Could you check a few things on this model? Use its own coordinates, in mm. Give positions to 0.01 mm unless a question says otherwise; leave off trailing zeros. Write each loop counter-clockwise with the first axis right and the second up, starting at its lowest first coordinate (ties: lowest second). Pieces come first, ordered by that corner, then holes. Notation, with made-up numbers: (59.5, -24) -> (72.5, -24) arc R23 ccw to (72.5, 6) -> close; hole circle Ø2 at (44, 44). An arc over 180 degrees is marked (long way). One line per question, with ' | ' between items.
from build123d import *

# Parameters (mm, degrees)
BASPROSKE_W         = 20
BASPROSKE_H         = 19.5
TOOTHCUT_DEPTH      = 35.066112194
TEETHCUTS_COUNT     = 11
BORSKE_R            = 2.5
BORE_DEPTH          = 50.0000508
SKETCH1_R           = 2.6
CUT_EXTRUDE1_DEPTH  = 35.008132728
BOSS_EXTRUDE1_DEPTH = 20


with BuildPart() as part:
    # BasProSke → Base-Revolve (revolve)
    with BuildSketch(Plane(origin=(0, 0, 0), x_dir=(1, 0, 0), z_dir=(0, 1, 0)), mode=Mode.PRIVATE) as base_revolve_sk:
        with Locations((10, 9.75)):
            Rectangle(BASPROSKE_W, BASPROSKE_H)
    revolve(base_revolve_sk.sketch.rotate(Axis((-10, 0, 0), (1, 0, 0)), 180), axis=Axis((-10, 0, 0), (1, 0, 0)))

    # TooCutSke → ToothCut (cut, through all)
    with BuildSketch(Plane(origin=(0, 0, 0), x_dir=(0, 0, -1), z_dir=(1, 0, 0))):
        with BuildLine():
            ThreePointArc((1.981256207, 12.594110721), (0, 12.749), (-1.981256207, 12.594110721))
            ThreePointArc((-1.981256207, 12.594110721), (-2.46948003, 16.158725125), (-4.75478191, 18.937615852))
            ThreePointArc((-4.75478191, 18.937615852), (0, 19.5254), (4.75478191, 18.937615852))
            ThreePointArc((4.75478191, 18.937615852), (2.46948003, 16.158725125), (1.981256207, 12.594110721))
        make_face()
    toothcut = extrude(amount=TOOTHCUT_DEPTH, mode=Mode.SUBTRACT)

    # TeethCuts: ToothCut ×11 about axis
    teethcuts_axis = Axis((0, 0, 0), (1, 0, 0))
    for i in range(1, TEETHCUTS_COUNT):
        add(toothcut.rotate(teethcuts_axis, i * 360 / TEETHCUTS_COUNT), mode=Mode.SUBTRACT)

    # BorSke → Bore (cut, symmetric)
    with BuildSketch(Plane(origin=(0, 0, 0), x_dir=(0, 0, -1), z_dir=(1, 0, 0))):
        with Locations(Location((0, 0, 0), (0, 0, 180))):
            Circle(BORSKE_R)
    extrude(amount=BORE_DEPTH, both=True, mode=Mode.SUBTRACT)

    # Sketch1 → Cut-Extrude1 (cut, through all)
    with BuildSketch(Plane(origin=(20, 0, 0), x_dir=(0, 0, -1), z_dir=(1, 0, 0))):
        Circle(SKETCH1_R)
    extrude(amount=-CUT_EXTRUDE1_DEPTH, mode=Mode.SUBTRACT)

    # Sketch2 → Boss-Extrude1 (add, through all)
    with BuildSketch(Plane(origin=(20, 0, 0), x_dir=(0, 0, -1), z_dir=(1, 0, 0))):
        with BuildLine():
            Line((-1.600307301, 2.0491502), (1.599692663, 2.04963006))
            ThreePointArc((1.599692663, 2.04963006), (-0.000389886, 2.599999971), (-1.600307301, 2.0491502))
        make_face()
    extrude(amount=-BOSS_EXTRUDE1_DEPTH)


solid = part.part
Q1. Imagine slicing it at B-B on y = 8.5. Please give me the cut outline in (x, z).
Answer below:
outline: (0, -13.22) -> (20, -13.22) -> (20, 13.22) -> (0, 13.22) -> close
Q2. Imagine slicing it at C-C on z = 7.5. Please give me the cut outline in (x, y).
Answer below:
outline: (0, -15.42) -> (20, -15.42) -> (20, 10.31) -> (0, 10.31) -> close
Q3. Will these pins go through, and if not, where does the flat tip stop? pin 1 (4.5 mm diameter, centred on y = 0, z = 0, fed in from -X); pin 2 (12 mm diameter, centred on x = 6.5, y = 3.5, fed in from +Z); pin 3 (10 mm diameter, centred on x = 7, z = -12, fed in from +Y); pin 4 (3 mm diameter, centred on x = 2.5, z = 2, fed in from +Y).
Answer below:
pin 1: stops at x = 0 | pin 2: stops at z = 19.4 | pin 3: stops at y = 13.36 | pin 4: stops at y = 17.8
Q4. If I drill on line 1 along Y through (x, z) = (12.5, 0); line 2 along Y through (x, z) = (10.75, 17); line 3 along Z through (x, y) = (6.25, -1.5), over which ranges is the centre line in solid material (lowest first)?
Answer below:
line 1: y = -19.5 to -2.6, 2.05 to 12.75 | line 2: y = -8.9 to -5.86, 0.36 to 4.36 | line 3: z = -12.66 to -2.12, 2.12 to 12.66
Q5. If we mould it in two halves opening along Z, with no side actions, what happens to faces 1 (the cylindrical face through (9.86, 0.127, -16.28)), 2 (the cylindrical face through (9.86, -16.23, -2.18)), 3 (the flat face through (0, 4, 0)), 4 (the cylindrical face through (10.14, -16.4, 10.55))? For each: +Z half, -Z half, draft (parallel to the pull), parting line (faces both ways), or undercut.
Answer below:
face 1: undercut | face 2: undercut | face 3: draft | face 4: +Z half
Q6. Imagine slicing it at A-A on z = 0. Please give me the cut outline in (x, y), and give its area (3 significant figures).
Answer below:
outline: (0, -19.5) -> (20, -19.5) -> (20, -2.6) -> (0, -2.6) -> close; (0, 2.05) -> (20, 2.05) -> (20, 12.75) -> (0, 12.75) -> close | area: 552 mm^2
